Can you work these out from the model? Positions are in its coordinate system, mm. A direction names the side the tool comes from. Give positions to 0.01 mm unless a question says otherwise; leave off trailing zeros. Loops run counter-clockwise (first coordinate to the right, second up) from the corner with the lowest first, then second, coordinate; pieces in that order, holes last. Notation, with made-up numbers: (37, -6.75) -> (82, -6.75) arc R20 ccw to (82, 17.25) -> close; hole circle Ø6 at (-21, 3.25). An arc over 180 degrees is marked (long way). One line per question, with ' | ' between items.
from build123d import *

# Parameters (mm, degrees)
SKETCH_1_W          = 5
SKETCH_1_H          = 10
EXTRUDE_1_DEPTH     = 240
SKETCH_3_R          = 5.5
CUT_EXTRUDE_1_DEPTH = 90
SKETCH_5_W          = 15
SKETCH_5_H          = 15
CUT_EXTRUDE_2_DEPTH = 80


with BuildPart() as part:
    # 草图1 → 凸台-拉伸1 (new body)
    with BuildSketch(Plane.XY):
        Polygon((0, -5), (0, 0), (-40, 0), (-40, 25), (-45, 25), (-45, -5), (-40, -5), align=None)
        Polygon((40, 25), (40, 0), (0, 0), (0, -5), (40, -5), (45, -5), (45, 25), align=None)
        with Locations((-42.5, -10)):
            Rectangle(SKETCH_1_W, SKETCH_1_H)
        with Locations((42.5, -10)):
            Rectangle(SKETCH_1_W, SKETCH_1_H)
    extrude(amount=EXTRUDE_1_DEPTH)

    # 草图3 → 切除-拉伸1 (cut, symmetric)
    with BuildSketch(Plane.ZY.offset(-40)):
        with Locations((30, -6)):
            Circle(SKETCH_3_R)
        with Locations((60, -6)):
            Circle(SKETCH_3_R)
        with Locations((90, -6)):
            Circle(SKETCH_3_R)
        with Locations((120, -6)):
            Circle(SKETCH_3_R)
        with Locations((150, -6)):
            Circle(SKETCH_3_R)
        with Locations((180, -6)):
            Circle(SKETCH_3_R)
        with Locations((210, -6)):
            Circle(SKETCH_3_R)
        Polygon((240, -5), (230, -15), (240, -15), align=None)
    extrude(amount=CUT_EXTRUDE_1_DEPTH, both=True, mode=Mode.SUBTRACT)

    # 草图5 → 切除-拉伸2 (cut)
    with BuildSketch(Plane(origin=(-40, 0, 0), x_dir=(0, 0, -1), z_dir=(1, 0, 0))):
        with Locations((-210, -5)):
            Rectangle(SKETCH_5_W, SKETCH_5_H)
        with Locations((-180, -5)):
            Rectangle(SKETCH_5_W, SKETCH_5_H)
        with Locations((-150, -5)):
            Rectangle(SKETCH_5_W, SKETCH_5_H)
        with Locations((-120, -5)):
            Rectangle(SKETCH_5_W, SKETCH_5_H)
        with Locations((-90, -5)):
            Rectangle(SKETCH_5_W, SKETCH_5_H)
        with Locations((-60, -5)):
            Rectangle(SKETCH_5_W, SKETCH_5_H)
        with Locations((-30, -5)):
            Rectangle(SKETCH_5_W, SKETCH_5_H)
    extrude(amount=CUT_EXTRUDE_2_DEPTH, mode=Mode.SUBTRACT)


solid = part.part
Q1. If we section it at A-A (x = 22): State how many separate pieces and enclosed holes the cut face has, plus the area to 3 significant figures.
Entries:
separate pieces: 8 | enclosed holes: 0 | area: 675 mm²
Q2. If we section it at D-D (z = 162.5): Write out the boundary of the cut face in (x, y).
Entries:
outline: (-45, -15) -> (-40, -15) -> (-40, -5) -> (40, -5) -> (40, -15) -> (45, -15) -> (45, 25) -> (40, 25) -> (40, 0) -> (-40, 0) -> (-40, 25) -> (-45, 25) -> close
Q3. If we section it at B-B (y = 20.5): Write out the boundary of the cut face in (x, z), plus the area to 3 significant figures.
Entries:
outline: (-45, 0) -> (-40, 0) -> (-40, 240) -> (-45, 240) -> close; (40, 0) -> (45, 0) -> (45, 240) -> (40, 240) -> close | area: 2,400 mm²
Q4. On a 3-axis mill with a long thin cutter (end or side, diameter ignored), from which of +Z, -Z, +X, -X, +Y, -Y can I reach the whole of each face in a straight line? I mean faces 1 (the face through (43, 25, 118)), 2 (the face through (1, 0, 105)), 3 (the face through (-1, -3, 142.5)), 4 (the face through (-1, -5, 75)). Say none if no direction works.
Entries:
face 1: +Z, -Z, +X, -X, +Y | face 2: +Z, -Z, +Y | face 3: +Y, -Y | face 4: +Z, -Z, -Y
Q5. For pin 1 Ø6 at (y, z) = (-3.5, 178) entering from +X; pin 2 Ø16.5 at (x, z) = (-16, 78.5) entering from +Y; pin 3 Ø4.5 at (x, z) = (7, 167.5) entering from -Y, each with a flat end and sliding along its axis, tell me the tip position at first contact or that it passes through.
Entries:
pin 1: x = 45 | pin 2: y = 0 | pin 3: y = -5
Q6. If we section it at C-C (z = 30): Write out the boundary of the cut face in (x, y).
Entries:
outline: (-45, -15) -> (-40, -15) -> (-40, -11.5) -> (-45, -11.5) -> close; (-45, -0.5) -> (-40, -0.5) -> (-40, 25) -> (-45, 25) -> close; (40, -15) -> (45, -15) -> (45, -11.5) -> (40, -11.5) -> close; (40, -0.5) -> (45, -0.5) -> (45, 25) -> (40, 25) -> close
Q7. If I drill on probe 1 along X at (y, z) = (23, 190.5); probe 2 along Y at (x, z) = (42.2, 120); probe 3 along Y at (x, z) = (-26, 18), over which ranges is the centre line in solid material (lowest first)? Write a range as from..to.
Entries:
probe 1: -45..-40, 40..45 | probe 2: -15..-11.5, -0.5..25 | probe 3: -5..0
Q8. If we mould it in two halves opening along X, with no side actions, what happens to faces 5 (the face through (-1, -3, 217.5)), 6 (the face through (45, 5, 118)), 7 (the face through (-42.465, -5.758, 24.505))? For each: pulls with the +X half, pulls with the -X half, needs draft (parallel to the pull), parting line crosses it, or undercut.
Entries:
face 5: undercut | face 6: pulls with the +X half | face 7: needs draft
